Geometry check sheet. Reference: drawing and pictorial views, mm from the part's lowest x, y, z. A direction names the side the tool comes from. Coordinates: 2 decimals unless noted, no trailing zeros. Order: outer loops, then holes, each group sorted by start corner. A loop starts at its lowest first (then second) coordinate and runs counter-clockwise, first axis right, second up. Notation, with made-up numbers: M 61,-20.75 L 119,-20.75 A21 cw 119,10.25 Z; hole C -15,34 d11. An arc over 180 degrees is marked long. Return JSON: item names as keys, results as strings.
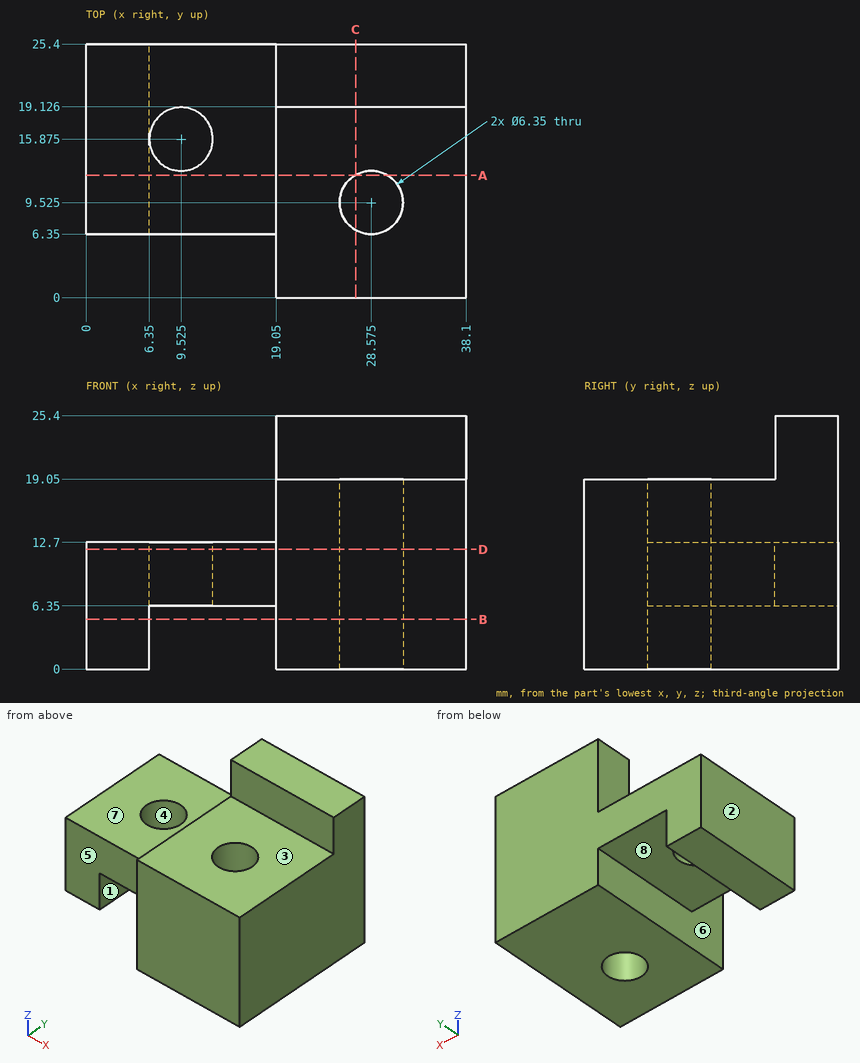
Q1. Cross-section at C-C, the plane x = 27. Record the boundary of the cut face in (y, z), and give its area (3 significant figures).
Values:
{"outline": "M 0,0 L 6.77,0 L 6.77,19.05 L 0,19.05 Z; M 12.28,0 L 25.4,0 L 25.4,25.4 L 19.13,25.4 L 19.13,19.05 L 12.28,19.05 Z", "area": "419 mm^2"}
Q2. Go/stop test with flat-tipped pins: pin 1 (15 mm diameter, centred on x = 33, y = 9, fed in from +Z); pin 2 (14 mm diameter, centred on x = 11.5, z = 8.5, fed in from -Y); pin 3 (8 mm diameter, centred on y = 21.5, z = 18, fed in from -X). Record where each tip stops, or that it passes through.
Values:
{"pin 1": "z = 19.05", "pin 2": "y = 6.35", "pin 3": "x = 19.05"}
Q3. Material ranges on line 1 along X through (y, z) = (9.5, 12.25); line 2 along X through (y, z) = (9.5, 19); line 3 along Z through (x, y) = (16.5, 23.25), recorded low to high.
Values:
{"line 1": "0 to 25.4, 31.75 to 38.1", "line 2": "19.05 to 25.4, 31.75 to 38.1", "line 3": "6.35 to 12.7"}
Q4. Draft check along X on the marked faces 1, 2, 3 and 4. Enter one of: pulls with the +X half, pulls with the -X half, needs draft (parallel to the pull), parting line crosses it, or undercut.
Values:
{"face 1": "undercut", "face 2": "pulls with the -X half", "face 3": "needs draft", "face 4": "undercut"}
Q5. Cross-section at B-B, the plane z = 5. Record the boundary of the cut face in (x, y) (3 decimals).
Values:
{"outline": "M 0,6.35 L 6.35,6.35 L 6.35,25.4 L 0,25.4 Z; M 19.05,0 L 38.1,0 L 38.1,25.4 L 19.05,25.4 Z; hole C 28.575,9.525 d6.35"}
Q6. Cross-section at A-A, the plane y = 12.25. Record the boundary of the cut face in (x, z), and give its area (3 significant figures).
Values:
{"outline": "M 0,0 L 6.35,0 L 6.35,6.35 L 19.05,6.35 L 19.05,0 L 26.95,0 L 26.95,19.05 L 19.05,19.05 L 19.05,12.7 L 0,12.7 Z; M 30.2,0 L 38.1,0 L 38.1,19.05 L 30.2,19.05 Z", "area": "462 mm^2"}
Q7. Cross-section at D-D, the plane z = 12. Record the boundary of the cut face in (x, y) (3 decimals).
Values:
{"outline": "M 0,6.35 L 19.05,6.35 L 19.05,0 L 38.1,0 L 38.1,25.4 L 0,25.4 Z; hole C 9.525,15.875 d6.35; hole C 28.575,9.525 d6.35"}
Q8. Tool access check on the marked faces 5, 6, 7 and 8. Record the directions out of +Z, -Z, +X, -X, +Y, -Y that give a thin tool (end or side, any length) a straight path to the whole face; none if there is none.
Values:
{"face 5": "+Z, -Z, -X, -Y", "face 6": "-Y", "face 7": "+Z, -X, +Y, -Y", "face 8": "-Z, +Y, -Y"}
